```python
from build123d import *

# Parameters (mm, degrees)
BOSS_EXTRUDE1_DEPTH                                  = 20
CBORE_FOR_M12_HEX_SOCKET_HEAD_CAP_SCREW1_D           = 13.5
CBORE_FOR_M12_HEX_SOCKET_HEAD_CAP_SCREW1_CBORE_D     = 20
CBORE_FOR_M12_HEX_SOCKET_HEAD_CAP_SCREW1_CBORE_DEPTH = 12.6
CBORE_FOR_M12_HEX_SOCKET_HEAD_CAP_SCREW2_D           = 13.5
CBORE_FOR_M12_HEX_SOCKET_HEAD_CAP_SCREW2_CBORE_D     = 20
CBORE_FOR_M12_HEX_SOCKET_HEAD_CAP_SCREW2_CBORE_DEPTH = 12.6
FILLET1_R                                            = 10
CHAMFER1_SIZE                                        = 1
CHAMFER2_SIZE                                        = 1


with BuildPart() as part:
    # Sketch1 → Boss-Extrude1 (new, symmetric)
    with BuildSketch(Plane(origin=(0, 0, 0), x_dir=(0, 0, -1), z_dir=(1, 0, 0))):
        Polygon((0, 0), (250, 0), (250, 750), (200, 750), (200, 675), (75, 50), (0, 50), align=None)
    extrude(amount=BOSS_EXTRUDE1_DEPTH, both=True)

    # CBORE for M12 Hex Socket Head Cap Screw1 (through all)
    with Locations(Plane(origin=(0, 50, 0), x_dir=(1, 0, 0), z_dir=(0, 1, 0))):
        with Locations((0, 55), (0, 20)):
            CounterBoreHole(CBORE_FOR_M12_HEX_SOCKET_HEAD_CAP_SCREW1_D / 2, CBORE_FOR_M12_HEX_SOCKET_HEAD_CAP_SCREW1_CBORE_D / 2, CBORE_FOR_M12_HEX_SOCKET_HEAD_CAP_SCREW1_CBORE_DEPTH)

    # CBORE for M12 Hex Socket Head Cap Screw2 (through all)
    with Locations(Plane.XY.offset(-200)):
        with Locations((0, 730), (0, 695)):
            CounterBoreHole(CBORE_FOR_M12_HEX_SOCKET_HEAD_CAP_SCREW2_D / 2, CBORE_FOR_M12_HEX_SOCKET_HEAD_CAP_SCREW2_CBORE_D / 2, CBORE_FOR_M12_HEX_SOCKET_HEAD_CAP_SCREW2_CBORE_DEPTH)

    # Fillet1
    fillet1_edges = [part.edges().sort_by_distance(p)[0] for p in [
        (0, 50, -75),
        (0, 675, -200),
    ]]
    fillet(fillet1_edges, radius=FILLET1_R)

    # Chamfer1
    chamfer1_edges = [part.edges().sort_by_distance(p)[0] for p in [
        (-20, 25, 0),
        (0, 50, 0),
        (20, 375, -250),
        (0, 750, -200),
        (0, 750, -250),
        (0, 0, -250),
        (0, 0, 0),
        (20, 750, -225),
        (20, 712.995097568, -200),
        (6.75, 0, -20),
        (6.75, 0, -55),
        (6.75, 695, -250),
        (6.75, 730, -250),
        (20, 25, 0),
        (-20, 50, -33.400980486),
        (20, 50, -33.400980486),
        (-20, 366.033936217, -138.206787243),
        (20, 366.033936217, -138.206787243),
        (-20, 52.266578587, -73.141850029),
        (20, 52.266578587, -73.141850029),
        (-20, 675.004818956, -199.951333267),
        (20, 675.004818956, -199.951333267),
        (-20, 712.995097568, -200),
        (-20, 750, -225),
        (20, 0, -125),
        (-20, 375, -250),
        (-20, 0, -125),
    ]]
    chamfer(chamfer1_edges, length=CHAMFER1_SIZE)

    # Chamfer2
    chamfer2_edges = [part.edges().sort_by_distance(p)[0] for p in [
        (-10, 50, -20),
        (-10, 50, -55),
        (-10, 695, -200),
        (-10, 730, -200),
    ]]
    chamfer(chamfer2_edges, length=CHAMFER2_SIZE)


solid = part.part
```
Geometry check sheet. Reference: the model listing, model coordinates, mm. A direction names the side the tool comes from. Coordinates: 2 decimals unless noted, no trailing zeros. Order: outer loops, then holes, each group sorted by start corner. A loop starts at its lowest first (then second) coordinate and runs counter-clockwise, first axis right, second up. Notation, with made-up numbers: (-13, 33) - (-7, 33) arc R12 cw to (-7, 39) - close; hole circle Ø10 at (84, -38). An arc over 180 degrees is marked (long way). Answer in a Markdown table with one row per item. Add a question column.
1. Section check D-D (x = 0). Give the number of separate pieces and of enclosed holes in the cut face, plus the area to 3 significant figures.
2. Gauge pin test, flat ends, axial feed: pin 1 Ø22 at (x, y) = (1.5, 690.5) entering from +Z; pin 2 Ø16 at (x, y) = (0, 730) entering from +Z; pin 3 Ø16 at (x, z) = (-3, -59.5) entering from +Y. Record the tip position at first contact, or that the pin passes through.
3. Material ranges on L1, parallel to Y at x = 0, z = -210; L2, parallel to Z at x = 0, y = 46; L3, parallel to X at y = 730, z = -235, recorded low to high. Write a range as [from, to].
4. Section check C-C (z = -134). Enter the section's corners in (x, y), plus the area to 3 significant figures.
5. Section check A-A (y = 695). Enter the section's corners in (x, z), plus the area to 3 significant figures.
6. Access from +Z, -Z, +X, -X, +Y, -Y to the whole of each face (thin tool, end or side, straight path). Record for faces 1 (the face through (0, 0, -123)), 2 (the face through (-2.17, 43.28, -45.24)).
7. Draft check along X on faces 3 (the face through (1.46, 723.41, -231.05)), 4 (the face through (0, 50, -34)), 5 (the face through (-20, 297, -178)), 6 (the face through (2, 723, -212.6)). Enter one of: +X half, -X half, draft (parallel to the pull), parting line (faces both ways), or undercut.
8. Section check B-B (z = -20). Enter the section's corners in (x, y).
Data:
| question | item | result |
|---|---|---|
| 1 | separate pieces | 5 |
| 1 | enclosed holes | 0 |
| 1 | area | 83,500 mm² |
| 2 | pin 1 | stops at z = -200 |
| 2 | pin 2 | stops at z = -212.6 |
| 2 | pin 3 | stops at y = 50.02 |
| 3 | L1 | y = [0, 685], [705, 720], [740, 750] |
| 3 | L2 | z = [-250, -65], [-45, -30], [-10, 0] |
| 3 | L3 | x = [-20, -6.75], [6.75, 20] |
| 4 | outline | (-20, 1) - (-19, 0) - (19, 0) - (20, 1) - (20, 339.9) - (19, 345) - (-19, 345) - (-20, 339.9) - close |
| 4 | area | 13,800 mm² |
| 5 | outline | (-20, -249) - (-19, -250) - (-7.75, -250) - (-6.75, -249) - (-6.75, -212.6) - (-10, -212.6) - (-10, -201) - (-11, -200) - (-19, -200) - (-20, -201) - close; (6.75, -249) - (7.75, -250) - (19, -250) - (20, -249) - (20, -201) - (19, -200) - (11, -200) - (10, -201) - (10, -212.6) - (6.75, -212.6) - close |
| 5 | area | 1,240 mm² |
| 6 | face 1 | +Z, -Z, +X, -X, -Y |
| 6 | face 2 | +Y |
| 7 | face 3 | undercut |
| 7 | face 4 | draft |
| 7 | face 5 | -X half |
| 7 | face 6 | undercut |
| 8 | outline | (-20, 1) - (-19, 0) - (-7.75, 0) - (-6.75, 1) - (-6.75, 37.4) - (-10, 37.4) - (-10, 49) - (-11, 50) - (-19, 50) - (-20, 49) - close; (6.75, 1) - (7.75, 0) - (19, 0) - (20, 1) - (20, 49) - (19, 50) - (11, 50) - (10, 49) - (10, 37.4) - (6.75, 37.4) - close |
